The drawing under review shows one solid part. Ordinate dimensions are in mm from its lowest x, y, z. A direction names the side the tool comes from. Give positions to 0.01 mm unless a question says otherwise; leave off trailing zeros. Loops run counter-clockwise (first coordinate to the right, second up) from the corner with the lowest first, then second, coordinate; pieces in that order, holes last. Notation, with made-up numbers: (-14.5, 56.5) - (18.5, 56.5) arc R29 cw to (18.5, 85.5) - close; hole circle Ø3 at (57.25, 80.25). An arc over 180 degrees is marked (long way). Return JSON: item names as keys, results as strings. Group by question number.
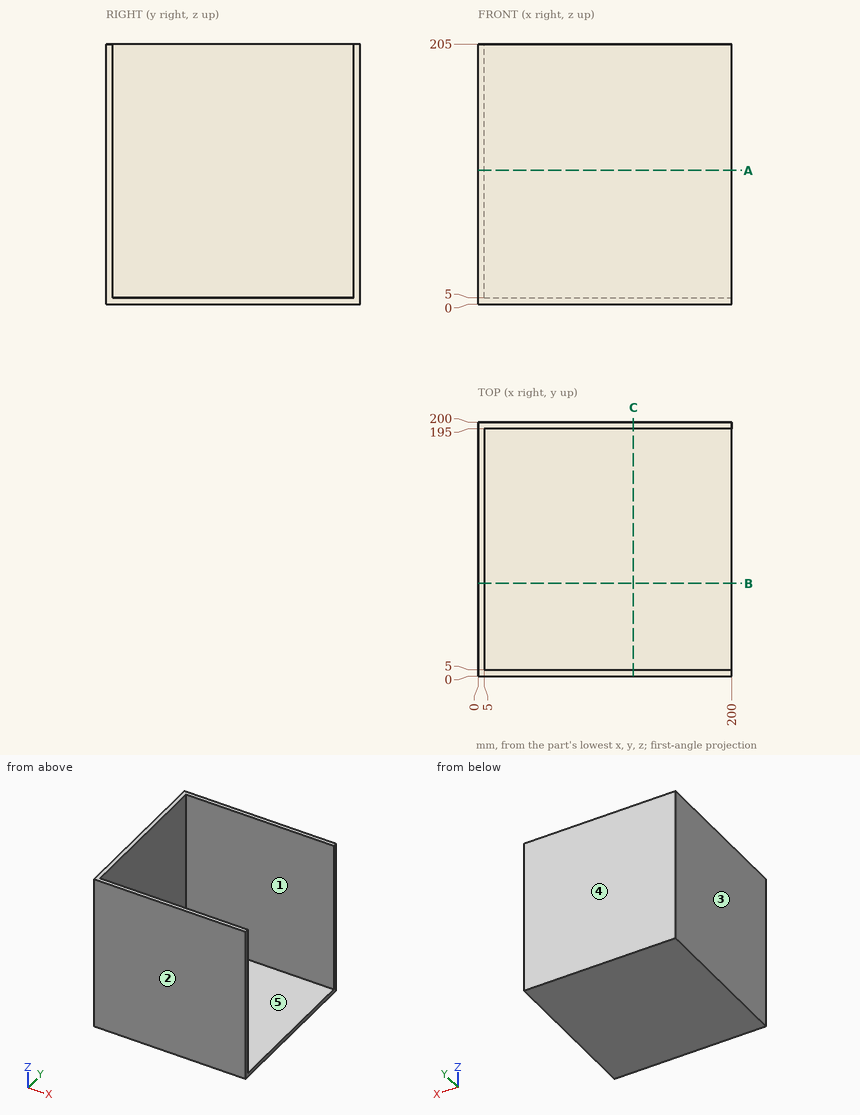
1) We need section A-A, the plane z = 105.5. Write out the cut boundary in (x, y), plus the area to 3 significant figures.
2) Tool access review of the marked faces 1 and 2: name each direction out of +Z, -Z, +X, -X, +Y, -Y from which nothing blocks a thin tool from reaching the whole face with its end or side.
3) To check wall thickness, follow line 1 (Y direction, x = 113.5, z = 22); line 2 (Z direction, x = 154, y = 143.5). State the ranges of each line that lie inside material, in increasing order.
4) Draft analysis for pull direction Y (two halves, no side actions). For the marked faces 3, 4 and 5, state which applies: +Y half, -Y half, draft (parallel to the pull), parting line (faces both ways), or undercut.
5) We need section C-C, the plane x = 122.5. Write out the cut boundary in (y, z).
6) For pin 1 Ø3 at (x, y) = (123, 58.5) entering from -Z; pin 2 Ø5 at (x, y) = (147.5, 178.5) entering from +Z; pin 3 Ø12 at (y, z) = (124, 127) entering from +X, all flat-tipped, find the tip position at first contact; note any pin that passes through.
7) We need section B-B, the plane y = 73. Write out the cut boundary in (x, z).
Findings:
{
 "1": {"outline": "(0, 0) - (200, 0) - (200, 5) - (5, 5) - (5, 195) - (200, 195) - (200, 200) - (0, 200) - close", "area": "2,950 mm^2"},
 "2": {"face 1": "+Z, +X", "face 2": "+Z, -Z, +X, -X, -Y"},
 "3": {"line 1": "y = 0 to 5, 195 to 200", "line 2": "z = 0 to 5"},
 "4": {"face 3": "draft", "face 4": "+Y half", "face 5": "undercut"},
 "5": {"outline": "(0, 0) - (200, 0) - (200, 205) - (195, 205) - (195, 5) - (5, 5) - (5, 205) - (0, 205) - close"},
 "6": {"pin 1": "stops at z = 0", "pin 2": "stops at z = 5", "pin 3": "stops at x = 5"},
 "7": {"outline": "(0, 0) - (200, 0) - (200, 5) - (5, 5) - (5, 205) - (0, 205) - close"}
}
